```python
from build123d import *

# Parameters (mm, degrees)
SKETCH1_W                                            = 30
SKETCH1_H                                            = 113
BOSS_EXTRUDE1_DEPTH                                  = 90
SKETCH3_W                                            = 95
SKETCH3_H                                            = 45.23
CUT_EXTRUDE1_DEPTH                                   = 90
SKETCH4_W                                            = 30
SKETCH4_H                                            = 10
CUT_EXTRUDE2_DEPTH                                   = 10
F_5_0_5_DIAMETER_HOLE1_D                             = 5
F_5_0_5_DIAMETER_HOLE1_DEPTH                         = 6.497848452
F_5_0_5_DIAMETER_HOLE1_CSINK_D                       = 5.05
F_5_0_5_DIAMETER_HOLE1_CSINK_ANGLE                   = 90
F_5_0_5_DIAMETER_HOLE1_TIP                           = 1.502151548
SKETCH9_W                                            = 7
SKETCH9_H                                            = 17.5
BOSS_EXTRUDE2_DEPTH                                  = 3
CSK_FOR_M3_HEX_SOCKET_COUNTERSUNK_CAP_SC_D           = 3.2
CSK_FOR_M3_HEX_SOCKET_COUNTERSUNK_CAP_SC_DEPTH       = 7.23862301
CSK_FOR_M3_HEX_SOCKET_COUNTERSUNK_CAP_SC_CSINK_D     = 6.72
CSK_FOR_M3_HEX_SOCKET_COUNTERSUNK_CAP_SC_CSINK_ANGLE = 90
CSK_FOR_M3_HEX_SOCKET_COUNTERSUNK_CAP_SC_TIP         = 0.96137699
SKETCH14_W                                           = 7
SKETCH14_H                                           = 17.5
BOSS_EXTRUDE3_DEPTH                                  = 3
CSK_FOR_M3_HEX_SOCKET_COUNTERSUNK_CA_2_D             = 3.2
CSK_FOR_M3_HEX_SOCKET_COUNTERSUNK_CA_2_DEPTH         = 7.23862301
CSK_FOR_M3_HEX_SOCKET_COUNTERSUNK_CA_2_CSINK_D       = 6.72
CSK_FOR_M3_HEX_SOCKET_COUNTERSUNK_CA_2_CSINK_ANGLE   = 90
CSK_FOR_M3_HEX_SOCKET_COUNTERSUNK_CA_2_TIP           = 0.96137699


with BuildPart() as part:
    # Sketch1 → Boss-Extrude1 (new body)
    with BuildSketch(Plane(origin=(0, 0, 0), x_dir=(1, 0, 0), z_dir=(0, 1, 0))):
        Rectangle(SKETCH1_W, SKETCH1_H)
    extrude(amount=BOSS_EXTRUDE1_DEPTH)

    # Sketch3 → Cut-Extrude1 (cut)
    with BuildSketch(Plane(origin=(0, 0, 0), x_dir=(0, 0, -1), z_dir=(1, 0, 0))):
        with Locations((0, 62.385)):
            Rectangle(SKETCH3_W, SKETCH3_H)
    extrude(amount=-CUT_EXTRUDE1_DEPTH, mode=Mode.SUBTRACT)

    # Sketch4 → Cut-Extrude2 (cut)
    with BuildSketch(Plane(origin=(15, 0, 0), x_dir=(0, 0, -1), z_dir=(1, 0, 0))):
        with Locations((0, 5)):
            Rectangle(SKETCH4_W, SKETCH4_H)
    extrude(amount=-CUT_EXTRUDE2_DEPTH, mode=Mode.SUBTRACT)

    # Ø5.0 (5) Diameter Hole1
    with Locations(Plane(origin=(0, 39.77, 0), x_dir=(1, 0, 0), z_dir=(0, 1, 0))):
        with Locations((-8.5, 23.38), (-8.5, -18.62)):
            CounterSinkHole(F_5_0_5_DIAMETER_HOLE1_D / 2, F_5_0_5_DIAMETER_HOLE1_CSINK_D / 2, depth=F_5_0_5_DIAMETER_HOLE1_DEPTH, counter_sink_angle=F_5_0_5_DIAMETER_HOLE1_CSINK_ANGLE)
            with Locations((0, 0, -(F_5_0_5_DIAMETER_HOLE1_DEPTH + F_5_0_5_DIAMETER_HOLE1_TIP / 2))):  # 118° drill point
                Cone(0, F_5_0_5_DIAMETER_HOLE1_D / 2, F_5_0_5_DIAMETER_HOLE1_TIP, mode=Mode.SUBTRACT)

    # Sketch9 → Boss-Extrude2 (add)
    with BuildSketch(Plane(origin=(0, 0, -56.5), x_dir=(-1, 0, 0), z_dir=(0, 0, -1))):
        with Locations((0, -2)):
            Rectangle(SKETCH9_W, SKETCH9_H)
    extrude(amount=BOSS_EXTRUDE2_DEPTH)

    # CSK for M3 Hex Socket Countersunk Cap Sc
    with Locations(Plane(origin=(0, 0, -59.5), x_dir=(-1, 0, 0), z_dir=(0, 0, -1))):
        with Locations((0, -7.25)):
            CounterSinkHole(CSK_FOR_M3_HEX_SOCKET_COUNTERSUNK_CAP_SC_D / 2, CSK_FOR_M3_HEX_SOCKET_COUNTERSUNK_CAP_SC_CSINK_D / 2, depth=CSK_FOR_M3_HEX_SOCKET_COUNTERSUNK_CAP_SC_DEPTH, counter_sink_angle=CSK_FOR_M3_HEX_SOCKET_COUNTERSUNK_CAP_SC_CSINK_ANGLE)
            with Locations((0, 0, -(CSK_FOR_M3_HEX_SOCKET_COUNTERSUNK_CAP_SC_DEPTH + CSK_FOR_M3_HEX_SOCKET_COUNTERSUNK_CAP_SC_TIP / 2))):  # 118° drill point
                Cone(0, CSK_FOR_M3_HEX_SOCKET_COUNTERSUNK_CAP_SC_D / 2, CSK_FOR_M3_HEX_SOCKET_COUNTERSUNK_CAP_SC_TIP, mode=Mode.SUBTRACT)

    # Sketch14 → Boss-Extrude3 (add)
    with BuildSketch(Plane.XY.offset(56.5)):
        with Locations((0, -1.75)):
            Rectangle(SKETCH14_W, SKETCH14_H)
    extrude(amount=BOSS_EXTRUDE3_DEPTH)

    # CSK for M3 Hex Socket Countersunk Ca 2
    with Locations(Plane.XY.offset(59.5)):
        with Locations((0, -7)):
            CounterSinkHole(CSK_FOR_M3_HEX_SOCKET_COUNTERSUNK_CA_2_D / 2, CSK_FOR_M3_HEX_SOCKET_COUNTERSUNK_CA_2_CSINK_D / 2, depth=CSK_FOR_M3_HEX_SOCKET_COUNTERSUNK_CA_2_DEPTH, counter_sink_angle=CSK_FOR_M3_HEX_SOCKET_COUNTERSUNK_CA_2_CSINK_ANGLE)
            with Locations((0, 0, -(CSK_FOR_M3_HEX_SOCKET_COUNTERSUNK_CA_2_DEPTH + CSK_FOR_M3_HEX_SOCKET_COUNTERSUNK_CA_2_TIP / 2))):  # 118° drill point
                Cone(0, CSK_FOR_M3_HEX_SOCKET_COUNTERSUNK_CA_2_D / 2, CSK_FOR_M3_HEX_SOCKET_COUNTERSUNK_CA_2_TIP, mode=Mode.SUBTRACT)


solid = part.part
```
Geometry check sheet. Reference: the model listing, model coordinates, mm. A direction names the side the tool comes from. Coordinates: 2 decimals unless noted, no trailing zeros. Write each loop counter-clockwise with the first axis right and the second up, starting at its lowest first coordinate (ties: lowest second). Pieces come first, ordered by that corner, then holes. Notation, with made-up numbers: M 30,-16 L 51,-16 A6 ccw 51,-12 Z; hole C 71.5,89 d2. An arc over 180 degrees is marked long. Use one line per item in the form item = value. Start each with the question number.
1) Section check D-D on z = -50.5. Enter the section's corners in (x, y), and give its area (3 significant figures).
2) Set-up check for faces 1 (the flat face through (0, -5, -56.5)), 2 (the flat face through (5, 5, 0)), 3 (the flat face through (-7, 62, 47.5)), 4 (the flat face through (0, 7, 58)), 5 (the cylindrical face through (-8.17, 36.46, -25.86)): record each of +Z, -Z, +X, -X, +Y, -Y from which the full face is reachable in a straight line by a thin tool's end or side.
3) Thickness scan on probe 1 along Z at (x, y) = (-8.5, 38.5); probe 2 along Y at (x, z) = (-5, 1.5); probe 3 along Z at (x, y) = (-5.5, 55.5). Record the ranges inside material, lowest first. Write a range as from..to.
4) Section check C-C on y = 36. Enter the section's corners in (x, z), and give its area (3 significant figures).
5) Go/stop test with flat-tipped pins: pin 1 Ø2.5 at (x, y) = (0, -7.25) entering from +Z; pin 2 Ø8 at (x, y) = (7, 37) entering from -Z; pin 3 Ø1 at (x, y) = (3, 69.5) entering from +Z; pin 4 Ø2.5 at (x, z) = (1, -58.5) entering from +Y. Record where each tip stops, or that it passes through.
6) Section check A-A on y = 55. Enter the section's corners in (x, z), and give its area (4 significant figures).
7) Section check B-B on z = 28. Enter the section's corners in (x, y).
8) Release check for a two-part mould opening along X. For faces 6 (the flat face through (0, 63, 1)), 7 (the conical face through (-8.59, 32.03, -22.96)), 8 (the flat face through (10, 10, 0)) record: pulls with the +X half, pulls with the -X half, needs draft (parallel to the pull), parting line crosses it, or undercut.
Responses:
q1.outline = M -15,0 L 15,0 L 15,90 L -15,90 Z
q1.area = 2,700 mm2
q2.face_1 = +X, -X, -Y
q2.face_2 = +X, -Y
q2.face_3 = -X
q2.face_4 = +Z, +X, -X, +Y
q2.face_5 = none
q3.probe_1 = -56.5..-25.88, -20.88..16.12, 21.12..56.5
q3.probe_2 = 0..39.77, 85..90
q3.probe_3 = -56.5..-47.5, 47.5..56.5
q4.outline = M -15,-56.5 L 15,-56.5 L 15,56.5 L -15,56.5 Z; hole C -8.5,-23.38 d5; hole C -8.5,18.62 d5
q4.area = 3,350 mm2
q5.pin_1 = through
q5.pin_2 = -56.5
q5.pin_3 = 56.5
q5.pin_4 = 6.75
q6.outline = M -15,-56.5 L 15,-56.5 L 15,56.5 L -15,56.5 L -15,47.5 L 0,47.5 L 0,-47.5 L -15,-47.5 Z
q6.area = 1,965 mm2
q7.outline = M -15,0 L 15,0 L 15,90 L -15,90 L -15,85 L 0,85 L 0,39.77 L -15,39.77 Z
q8.face_6 = pulls with the -X half
q8.face_7 = undercut
q8.face_8 = needs draft
